Check sheet for the modelled part. Datum: model origin and axes. Units: mm. A direction names the side the tool comes from. Coordinates: 2 decimals unless noted, no trailing zeros. Loops run counter-clockwise (first coordinate to the right, second up) from the corner with the lowest first, then second, coordinate; pieces in that order, holes last. Notation, with made-up numbers: M 12.5,64 L 61.5,64 A15 ccw 61.5,69 Z; hole C -26,-15 d7. An arc over 180 degrees is marked long. Return JSON: item names as keys, results as strings.
from build123d import *

# Parameters (mm, degrees)
SKETCH106_R   = 6.5
SKETCH106_R_2 = 5
PAD071_DEPTH  = 30
SKETCH107_R   = 6.5
PAD074_DEPTH  = 3
SKETCH108_R   = 6.5
PAD075_DEPTH  = 3


with BuildPart() as part:
    # Sketch106 → Pad071 (new body)
    with BuildSketch(Plane.YZ):
        Circle(SKETCH106_R)
        Circle(SKETCH106_R_2, mode=Mode.SUBTRACT)
    extrude(amount=PAD071_DEPTH)

    # Sketch107 (on Face3 of Pad071) → Pad074 (join)
    with BuildSketch(Plane(origin=(0, 0, 0), x_dir=(0, 1, 0), z_dir=(-1, 0, 0))):
        with BuildLine():
            Line((-12.5, 15), (12.5, 15))
            Line((12.5, 15), (12.5, 0))
            ThreePointArc((-12.5, 0), (0, -12.5), (12.5, 0))
            Line((-12.5, 0), (-12.5, 15))
        make_face()
        Circle(SKETCH107_R, mode=Mode.SUBTRACT)
    extrude(amount=-PAD074_DEPTH)

    # Sketch108 (on Face3 of Pad074) → Pad075 (join)
    with BuildSketch(Plane.YZ.offset(30)):
        with BuildLine():
            Line((-12.5, -15), (-12.5, 0))
            ThreePointArc((12.5, 0), (0, 12.5), (-12.5, 0))
            Line((12.5, 0), (12.5, -15))
            Line((12.5, -15), (-12.5, -15))
        make_face()
        Circle(SKETCH108_R, mode=Mode.SUBTRACT)
    extrude(amount=-PAD075_DEPTH)


with BuildPart() as part_1:
    # Body045 placement: moved
    add(part.part.moved(Location((-62, 0, 0))))


solid = part_1.part
1) Section check D-D on y = -5.75. Record the cut outline in (x, z).
Answers:
{"outline": "M -62,-15 L -59,-15 L -59,-3.03 L -35,-3.03 L -35,-15 L -32,-15 L -32,11.1 L -35,11.1 L -35,3.03 L -59,3.03 L -59,11.1 L -62,11.1 Z"}
2) Section check C-C on x = -39.25. Record the cut outline in (y, z), then the cut area to 3 significant figures.
Answers:
{"outline": "C 0,0 d13; hole C 0,0 d10", "area": "54.2 mm²"}
3) Section check B-B on z = -1. Record the cut outline in (x, y).
Answers:
{"outline": "M -62,-12.5 L -59,-12.5 L -59,-6.42 L -35,-6.42 L -35,-12.5 L -32,-12.5 L -32,-4.9 L -62,-4.9 Z; M -62,4.9 L -32,4.9 L -32,12.5 L -35,12.5 L -35,6.42 L -59,6.42 L -59,12.5 L -62,12.5 Z"}
4) Draft check along X on faces 1 (the face through (-35, 0, -7)), 2 (the face through (-32, 0, -7)), 3 (the face through (-59, 0, -8)), 4 (the face through (-47.21, -1.08, -4.88)). Enter one of: +X half, -X half, draft (parallel to the pull), parting line (faces both ways), or undercut.
Answers:
{"face 1": "undercut", "face 2": "+X half", "face 3": "undercut", "face 4": "draft"}
5) Set-up check for faces 5 (the face through (-47.168, -5.158, -3.955)), 6 (the face through (-61, -12.5, -7)): record each of +Z, -Z, +X, -X, +Y, -Y from which the full face is reachable in a straight line by a thin tool's end or side.
Answers:
{"face 5": "none", "face 6": "+Z, -Z, +X, -X, -Y"}
6) Scan lines: line 1 along X through (y, z) = (-11, 0.5); line 2 along Z through (x, y) = (-44, 0); line 3 along Z through (x, y) = (-51.5, 2). Record each from-to range of solid material in increasing order. Write a range as [from, to].
Answers:
{"line 1": "[-62, -59], [-35, -32]", "line 2": "[-6.5, -5], [5, 6.5]", "line 3": "[-6.18, -4.58], [4.58, 6.18]"}
7) Go/stop test with flat-tipped pins: pin 1 Ø9 at (y, z) = (0, 0) entering from -X; pin 2 Ø3 at (x, z) = (-45.5, 3.5) entering from +Y; pin 3 Ø3 at (x, z) = (-43, 0) entering from -Y. Record where each tip stops, or that it passes through.
Answers:
{"pin 1": "through", "pin 2": "y = 6.18", "pin 3": "y = -6.5"}
8) Section check A-A on y = 0. Record the cut outline in (x, z), then the cut area to 3 significant figures.
Answers:
{"outline": "M -62,-15 L -59,-15 L -59,-6.5 L -35,-6.5 L -35,-15 L -32,-15 L -32,-5 L -62,-5 Z; M -62,5 L -32,5 L -32,12.5 L -35,12.5 L -35,6.5 L -59,6.5 L -59,12.5 L -62,12.5 Z", "area": "177 mm²"}
